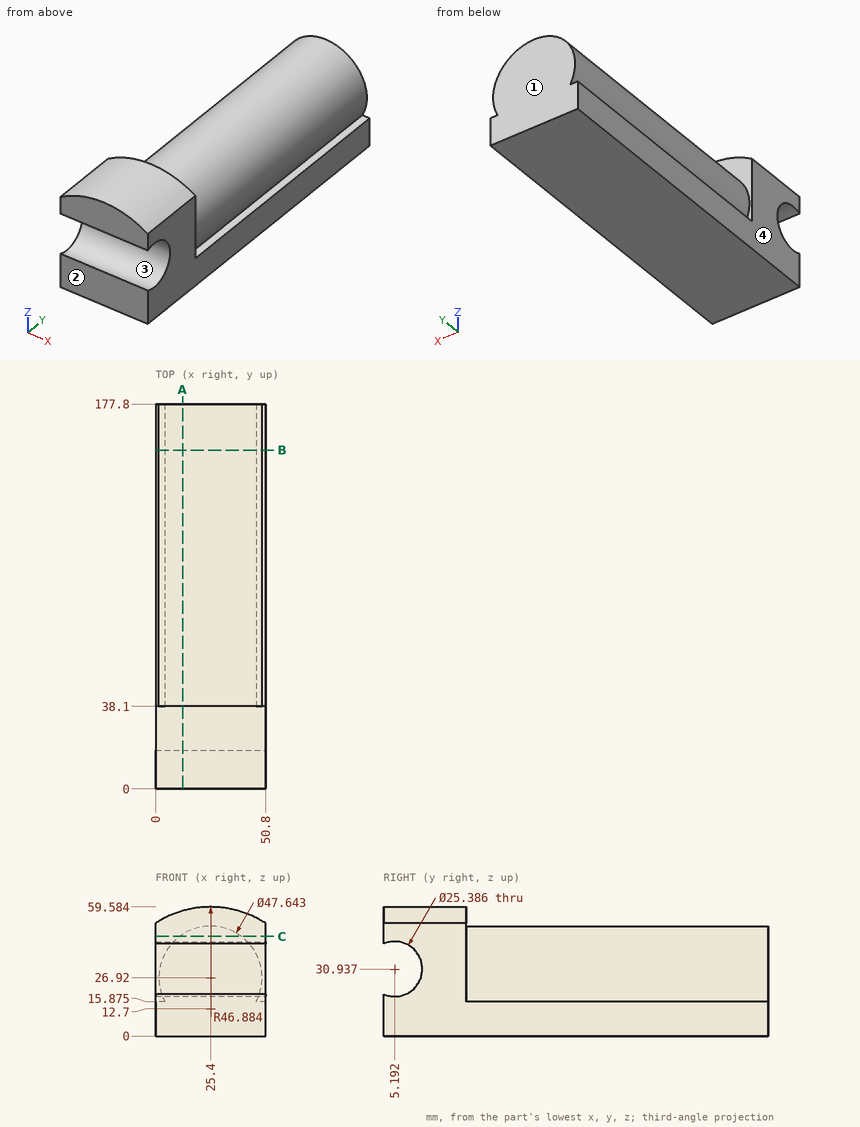
Design review of the part shown in the three views and the two pictorial views. Dimensions are in mm from the part's minimum x, y and z. Give positions to 0.01 mm unless a question says otherwise; leave off trailing zeros. Write each loop counter-clockwise with the first axis right and the second up, starting at its lowest first coordinate (ties: lowest second). Pieces come first, ordered by that corner, then holes. Notation, with made-up numbers: (-17.75, 10) - (-3.75, 10) arc R24 cw to (-3.75, 33) - close; hole circle Ø10 at (61, 68). An arc over 180 degrees is marked (long way). Return JSON: item names as keys, results as strings. Group by question number.
(1) We need section B-B, the plane y = 156.5. Give the boundary of the cut face in (x, z) (1 decimal), then the cut area to 3 significant figures.
(2) To check wall thickness, follow probe 1 along Y at (x, z) = (19, 53); probe 2 along Z at (x, y) = (25, 85); probe 3 along Z at (x, y) = (17, 160). State the ranges of each line that lie inside material, in increasing order.
(3) We need section C-C, the plane z = 46. Give the boundary of the cut face in (x, y), then the cut area to 3 significant figures.
(4) Mouldability with a two-part tool opening along Y and no side actions: class the marked faces 1, 2, 3 and 4 as +Y half, -Y half, draft (parallel to the pull), parting line (faces both ways), or undercut.
(5) Insertion check: pin 1 (5 mm diameter, centred on x = 34, y = 105, fed in from +Z); pin 2 (2 mm diameter, centred on y = 87.5, z = 29.5, fed in from +X); pin 3 (12 mm diameter, centred on y = 84, z = 35.5, fed in from +X); pin 4 (20.5 mm diameter, centred on y = 5.19, z = 30.94, fed in from -X). Each pin has a flat end and moves straight along its axis. Give the tip position at first contact, or say it passes through.
(6) We need section A-A, the plane x = 12.5. Give the boundary of the cut face in (y, z) (1 decimal).
Reported:
{
 "1": {"outline": "(0, 0) - (50.8, 0) - (50.8, 15.9) - (46.5, 15.9) arc R23.8 ccw (long way) to (4.3, 15.9) - (0, 15.9) - close", "area": "2,200 mm2"},
 "2": {"probe 1": "y = 0 to 38.1", "probe 2": "z = 0 to 50.74", "probe 3": "z = 0 to 49.21"},
 "3": {"outline": "(0, 0) - (50.8, 0) - (50.8, 38.1) - (39.66, 38.1) - (39.66, 177.8) - (11.14, 177.8) - (11.14, 38.1) - (0, 38.1) - close", "area": "5,920 mm2"},
 "4": {"face 1": "+Y half", "face 2": "-Y half", "face 3": "undercut", "face 4": "draft"},
 "5": {"pin 1": "stops at z = 49.95", "pin 2": "stops at x = 49.17", "pin 3": "stops at x = 49.08", "pin 4": "passes through"},
 "6": {"outline": "(0, 0) - (177.8, 0) - (177.8, 46.9) - (38.1, 46.9) - (38.1, 57.8) - (0, 57.8) - (0, 42.5) arc R12.7 cw (long way) to (0, 19.4) - close"}
}
